Check sheet for the modelled part. Datum: model origin and axes. Units: mm. Round coordinates to 2 decimals unless told otherwise and drop trailing zeros. Loops run counter-clockwise (first coordinate to the right, second up) from the corner with the lowest first, then second, coordinate; pieces in that order, holes last. Notation, with made-up numbers: (24.25, -30.5) - (74.25, -30.5) arc R8 cw to (74.25, -26.5) - close; hole circle Ø10 at (44.25, 13.25). An arc over 180 degrees is marked (long way). Put each result on its own line as item: value. Start each with the question number.
```python
from build123d import *

# Parameters (mm, degrees)
F1_DEPTH = 203.2
F2_R     = 50.8


with BuildPart() as f1:
    # F0 (on Top) → F1 (new body)
    with BuildSketch(Plane.XY):
        with BuildLine():
            ThreePointArc((0, -654.99996), (654.99996, 0), (0, 654.99996))
            Line((0, 654.99996), (0, -654.99996))
        make_face()
    extrude(amount=F1_DEPTH)

    # F2
    f2_edges = [f1.edges().sort_by_distance(p)[0] for p in [
        (654.99996, 0, 203.2),
        (654.99996, 0, 0),
        (0, 654.99996, 101.6),
        (0, -654.99996, 101.6),
    ]]
    fillet(f2_edges, radius=F2_R)


solid = f1.part
```
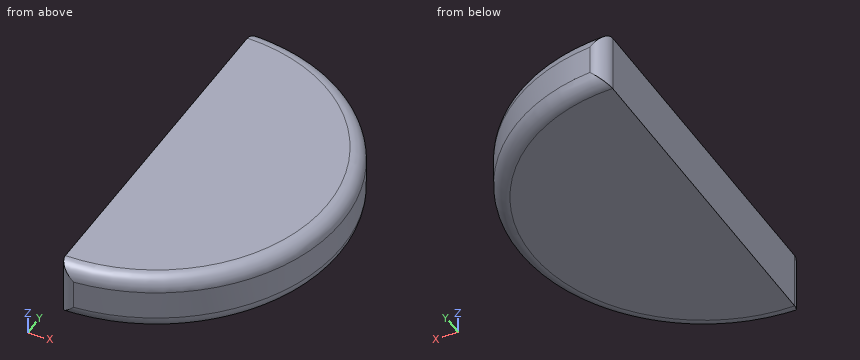
Q1. Material ranges on line 1 (X direction, y = -15.5, z = 85.5); line 2 (X direction, y = 19.5, z = 85); line 3 (Z direction, x = 424.5, y = 492), recorded low to high. Write a range as from..to.
Q2. Cross-section at B-B on z = 26. Enter the section's corners in (x, y).
Q3. Depth check by flat-ended pin: pin 1 Ø12 at (x, z) = (124.5, 82.5) entering from -Y; pin 2 Ø1.5 at (x, z) = (201.5, 67.5) entering from -Y; pin 3 Ø6 at (y, z) = (-252, 60.5) entering from +X (3 decimals). Enter the tip coordinate at first touch or a pass-through.
Q4. Cross-section at A-A on z = 114.5. Enter the section's corners in (x, y).
Answer list:
1. line 1: x = 0..654.82
1. line 2: x = 0..654.71
1. line 3: z = 28.45..174.75
2. outline: (0, -602.06) arc R50.8 ccw to (28.89, -647.89) arc R648.54 ccw to (28.89, 647.89) arc R50.8 ccw to (0, 602.06) - close
3. pin 1: stops at y = -644.19
3. pin 2: stops at y = -623.48
3. pin 3: stops at x = 605.825
4. outline: (0, -602.06) arc R50.8 ccw to (55.07, -652.68) arc R655 ccw to (55.07, 652.68) arc R50.8 ccw to (0, 602.06) - close
